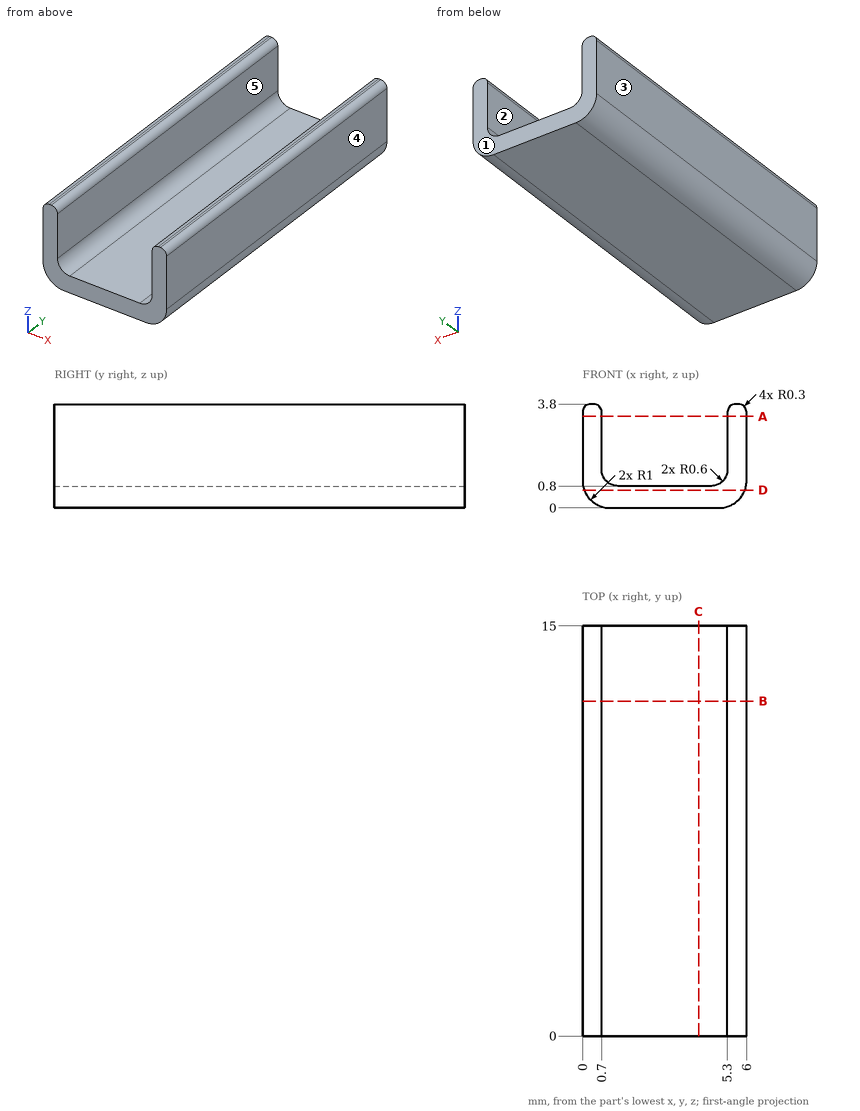
Geometry: see drawing. Coordinates: mm, zero at the bounding-box minimum. A direction names the side the tool comes from. Round coordinates to 2 decimals unless told otherwise and drop trailing zeros. Loops run counter-clockwise (first coordinate to the right, second up) from the corner with the lowest first, then second, coordinate; pieces in that order, holes last. Notation, with made-up numbers: (-39, -22.75) -> (-9, -22.75) arc R22 ccw to (-9, -16.75) -> close; hole circle Ø7 at (39.25, -39). An arc over 180 degrees is marked (long way). Use one line per item in the form item = value. Start each with the question number.
Item 1: Set-up query: the marked faces 1 and 2. Return all of +Z, -Z, +X, -X, +Y, -Y with unobstructed straight access to the full face (end or side cutting, diameter ignored); none if empty.
Item 2: Section query D-D on z = 0.65. Return the cut outline in (x, y).
Item 3: Mould query, pull axis X, two halves, no side actions, for the marked faces 3, 4 and 5. Classes: pulls with the +X half, pulls with the -X half, needs draft (parallel to the pull), parting line crosses it, or undercut.
Item 4: Section query A-A on z = 3.35. Return the cut outline in (x, y).
Item 5: Section query B-B on y = 12.25. Return the cut outline in (x, z).
Item 6: Contact query for flat-ended pins moving along their axis: pin 1 Ø1 at (x, z) = (4, 3) entering from +Y; pin 2 Ø2.5 at (x, y) = (2.5, 7.5) entering from +Z. Output: stop coordinate, or through.
Item 7: Material intervals for L1, parallel to X at y = 13, z = 1.65; L2, parallel to Z at x = 2, y = 14; L3, parallel to X at y = 7.75, z = 1.05, sorted ascending. Write a range as from..to.
Item 8: Section query C-C on x = 4.25. Return the cut outline in (y, z), then the cut area to 3 significant figures.
Ans:
q1.face_1 = +Z, -Z, +X, -X, +Y
q1.face_2 = +Z, +Y, -Y
q2.outline = (0.06, 0) -> (5.94, 0) -> (5.94, 15) -> (0.06, 15) -> close
q3.face_3 = pulls with the -X half
q3.face_4 = pulls with the +X half
q3.face_5 = undercut
q4.outline = (0, 0) -> (0.7, 0) -> (0.7, 15) -> (0, 15) -> close; (5.3, 0) -> (6, 0) -> (6, 15) -> (5.3, 15) -> close
q5.outline = (0, 1) arc R1 ccw to (1, 0) -> (5, 0) arc R1 ccw to (6, 1) -> (6, 3.5) arc R0.3 ccw to (5.7, 3.8) -> (5.6, 3.8) arc R0.3 ccw to (5.3, 3.5) -> (5.3, 1.4) arc R0.6 cw to (4.7, 0.8) -> (1.3, 0.8) arc R0.6 cw to (0.7, 1.4) -> (0.7, 3.5) arc R0.3 ccw to (0.4, 3.8) -> (0.3, 3.8) arc R0.3 ccw to (0, 3.5) -> close
q6.pin_1 = through
q6.pin_2 = 0.8
q7.L1 = 0..0.7, 5.3..6
q7.L2 = 0..0.8
q7.L3 = 0..0.81, 5.19..6
q8.outline = (0, 0) -> (15, 0) -> (15, 0.8) -> (0, 0.8) -> close
q8.area = 12.0 mm^2
